Design review of the part shown in the three views and the two pictorial views. Dimensions are in mm from the part's minimum x, y and z. A direction names the side the tool comes from. Coordinates: 2 decimals unless noted, no trailing zeros. Write each loop counter-clockwise with the first axis right and the second up, starting at its lowest first coordinate (ties: lowest second). Pieces come first, ordered by that corner, then holes. Notation, with made-up numbers: (51.5, -23.75) -> (82.5, -23.75) arc R28 cw to (82.5, 13.25) -> close; hole circle Ø9 at (4.25, -26). An arc over 180 degrees is marked (long way). Write item = value, one per line. Start each with the question number.
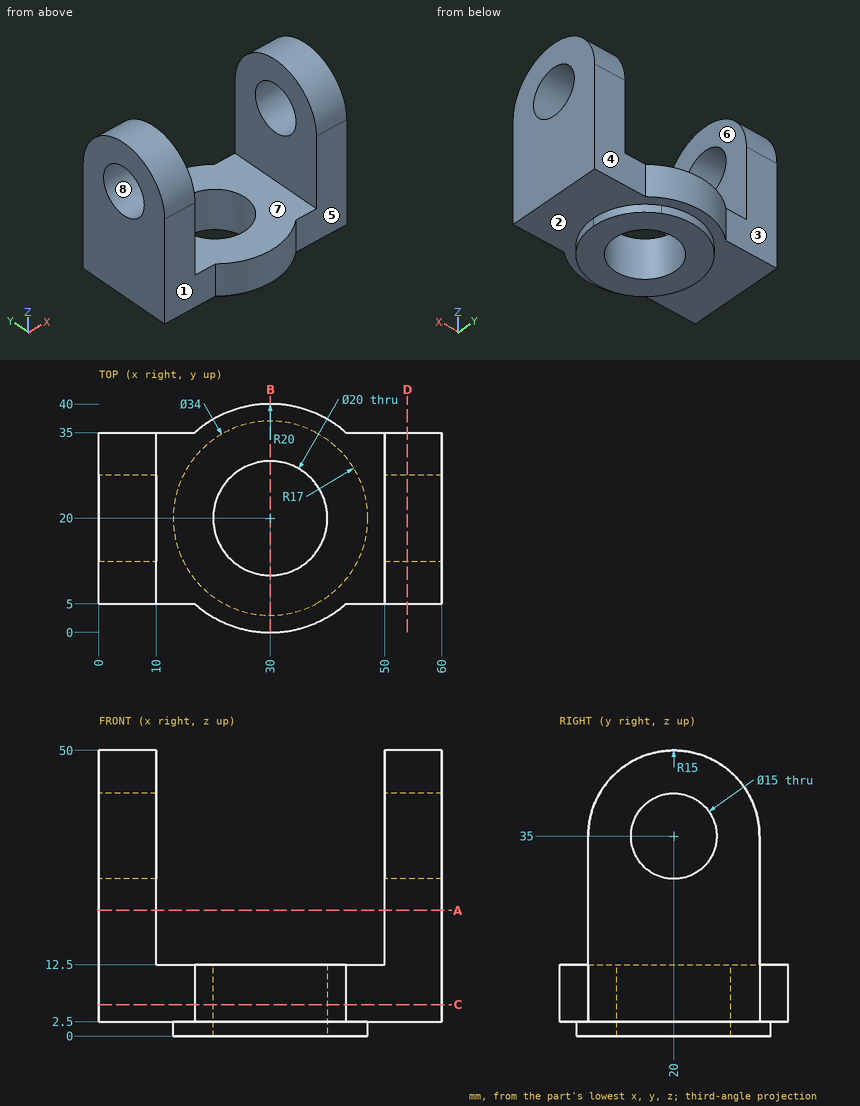
(1) Take a section at C-C, the plane z = 5.5. State the section outline as (x, y) points, then the cut area to 3 significant figures.
(2) For line 1 (Z direction, x = 6.5, y = 20); line 2 (X direction, y = 10.5, z = 28.5); line 3 (Y direction, x = 30, z = 7.25), list the stretches that pass through material, from the lowest coordinate up.
(3) For the marked faces 1, 2, 3, 4 and 5, list the 3-axis set-ups (+Z, -Z, +X, -X, +Y, -Y) from which the entire face can be reached by the end or side of a thin tool; tool diameter is ignored.
(4) Mouldability with a two-part tool opening along Z and no side actions: class the marked faces 6, 7 and 8 as pulls with the +Z half, pulls with the -Z half, needs draft (parallel to the pull), parting line crosses it, or undercut.
(5) Take a section at D-D, the plane x = 54. State the section outline as (y, z) points.
(6) For pin 1 Ø18.5 at (x, z) = (11.5, 23) entering from +Y; pin 2 Ø8.5 at (x, z) = (5.5, 18.5) entering from -Y, all flat-tipped, find the tip position at first contact; note any pin that passes through.
(7) Take a section at A-A, the plane z = 22. State the section outline as (x, y) points.
(8) Take a section at B-B, the plane x = 30. State the section outline as (y, z) points, then the cut area to 3 significant figures.
Report:
q1.outline = (0, 5) -> (16.77, 5) arc R20 ccw to (43.23, 5) -> (60, 5) -> (60, 35) -> (43.23, 35) arc R20 ccw to (16.77, 35) -> (0, 35) -> close; hole circle Ø20 at (30, 20)
q1.area = 1,670 mm2
q2.line_1 = 2.5 to 27.5, 42.5 to 50
q2.line_2 = 0 to 10, 50 to 60
q2.line_3 = 0 to 10, 30 to 40
q3.face_1 = +Z, -Z, -X, -Y
q3.face_2 = -Z
q3.face_3 = +Z, -Z, -X, +Y
q3.face_4 = +Z, -Z, +X, +Y
q3.face_5 = +Z, -Z, +X, -Y
q4.face_6 = needs draft
q4.face_7 = pulls with the +Z half
q4.face_8 = undercut
q5.outline = (5, 2.5) -> (35, 2.5) -> (35, 35) arc R15 ccw to (5, 35) -> close; hole circle Ø15 at (20, 35)
q6.pin_1 = 35
q6.pin_2 = 5
q7.outline = (0, 5) -> (10, 5) -> (10, 35) -> (0, 35) -> close; (50, 5) -> (60, 5) -> (60, 35) -> (50, 35) -> close
q8.outline = (0, 2.5) -> (3, 2.5) -> (3, 0) -> (10, 0) -> (10, 12.5) -> (0, 12.5) -> close; (30, 0) -> (37, 0) -> (37, 2.5) -> (40, 2.5) -> (40, 12.5) -> (30, 12.5) -> close
q8.area = 235 mm2
